Could you check a few things on this model? Use its own coordinates, in mm. A direction names the side the tool comes from. Give positions to 0.01 mm unless a question says otherwise; leave off trailing zeros. Write each question's results on one line, items separated by ' | '. Start each with the question number.
(1) For pin 1 (0.8 mm diameter, centred on x = 136, z = 14.5, fed in from +Y), with a flat end and sliding along its axis, tell me the tip position at first contact or that it passes through.
(2) Suppose I cut it at A-A (y = 12.5). Count the separate pieces of the cut face and the enclosed holes in it, and give its area (3 significant figures).
(3) If we mould it in two halves opening along X, with no side actions, what happens to faces 3 (the face through (233.054, 12.664, 12.522)), 4 (the face through (0, 5, 13)), 5 (the face through (46.364, 12.736, 12.522))? For each: released by +X, released by -X, zero draft, split by the parting line, or undercut.
(4) On a 3-axis mill with a long thin cutter (end or side, diameter ignored), from which of +Z, -Z, +X, -X, +Y, -Y can I reach the whole of each face in a straight line? I mean faces 1 (the face through (0.644, 12.736, 12.522)), 2 (the face through (99.704, 12.736, 12.522)). Say none if no direction works.
(5) I need wall thicknesses on line 1 (Y direction, x = 37.5, z = 24.5). Which ranges of the line are inside material? Lowest first, please.
from build123d import *

# Parameters (mm, degrees)
BOSS_EXTRUDE1_DEPTH = 25.4


with BuildPart() as part:
    # Sketch1 → Boss-Extrude1 (new body)
    with BuildSketch(Plane.XY):
        Polygon((0, 0), (233.68, 0), (233.68, 10.16), (232.41, 15.24), (229.87, 15.24), (228.6, 10.16), (226.06, 10.16), (224.79, 15.24), (222.25, 15.24), (220.98, 10.16), (218.44, 10.16), (217.17, 15.24), (214.63, 15.24), (213.36, 10.16), (210.82, 10.16), (209.55, 15.24), (207.01, 15.24), (205.74, 10.16), (203.2, 10.16), (201.93, 15.24), (199.39, 15.24), (198.12, 10.16), (195.58, 10.16), (194.31, 15.24), (191.77, 15.24), (190.5, 10.16), (187.96, 10.16), (186.69, 15.24), (184.15, 15.24), (182.88, 10.16), (180.34, 10.16), (179.07, 15.24), (176.53, 15.24), (175.26, 10.16), (172.72, 10.16), (171.45, 15.24), (168.91, 15.24), (167.64, 10.16), (165.1, 10.16), (163.83, 15.24), (161.29, 15.24), (160.02, 10.16), (157.48, 10.16), (156.21, 15.24), (153.67, 15.24), (152.4, 10.16), (149.86, 10.16), (148.59, 15.24), (146.05, 15.24), (144.78, 10.16), (142.24, 10.16), (140.97, 15.24), (138.43, 15.24), (137.16, 10.16), (134.62, 10.16), (133.35, 15.24), (130.81, 15.24), (129.54, 10.16), (127, 10.16), (125.73, 15.24), (123.19, 15.24), (121.92, 10.16), (119.38, 10.16), (118.11, 15.24), (115.57, 15.24), (114.3, 10.16), (111.76, 10.16), (110.49, 15.24), (107.95, 15.24), (106.68, 10.16), (104.14, 10.16), (102.87, 15.24), (100.33, 15.24), (99.06, 10.16), (96.52, 10.16), (95.25, 15.24), (92.71, 15.24), (91.44, 10.16), (88.9, 10.16), (87.63, 15.24), (85.09, 15.24), (83.82, 10.16), (81.28, 10.16), (80.01, 15.24), (77.47, 15.24), (76.2, 10.16), (73.66, 10.16), (72.39, 15.24), (69.85, 15.24), (68.58, 10.16), (66.04, 10.16), (64.77, 15.24), (62.23, 15.24), (60.96, 10.16), (58.42, 10.16), (57.15, 15.24), (54.61, 15.24), (53.34, 10.16), (50.8, 10.16), (49.53, 15.24), (46.99, 15.24), (45.72, 10.16), (43.18, 10.16), (41.91, 15.24), (39.37, 15.24), (38.1, 10.16), (35.56, 10.16), (34.29, 15.24), (31.75, 15.24), (30.48, 10.16), (27.94, 10.16), (26.67, 15.24), (24.13, 15.24), (22.86, 10.16), (20.32, 10.16), (19.05, 15.24), (16.51, 15.24), (15.24, 10.16), (12.7, 10.16), (11.43, 15.24), (8.89, 15.24), (7.62, 10.16), (5.08, 10.16), (3.81, 15.24), (1.27, 15.24), (0, 10.16), align=None)
    extrude(amount=BOSS_EXTRUDE1_DEPTH)


solid = part.part
Output values:
1) pin 1: y = 10.16
2) separate pieces: 31 | enclosed holes: 0 | area: 3,080 mm2
3) face 3: released by +X | face 4: released by -X | face 5: undercut
4) face 1: +Z, -Z, -X, +Y | face 2: +Z, -Z, +Y
5) line 1: 0 to 10.16
